Read the model definition and answer for the solid it produces. Units are mm, in the model's axes. Give positions to 0.01 mm unless a question says otherwise; leave off trailing zeros. Loops run counter-clockwise (first coordinate to the right, second up) from the corner with the lowest first, then second, coordinate; pieces in that order, holes last. Notation, with made-up numbers: (15.25, -32.5) - (50.25, -32.5) arc R16 ccw to (50.25, -28.5) - close; hole circle Ø5 at (-30, -28). An arc over 180 degrees is marked (long way). Write item = value, one per line. Start each with the question number.
Autodesk Inventor part; units mm, degrees
ref_plane "YZ Plane" through (0, 0, 0) normal (1, 0, 0) x (0, 1, 0)
ref_plane "XZ Plane" through (0, 0, 0) normal (0, 1, 0) x (-1, 0, 0)
ref_plane "XY Plane" through (0, 0, 0) normal (0, 0, 1) x (1, 0, 0)
sketch "Sketch1" plane through (0, 0, 0) normal (0, 1, 0) x (-1, 0, 0)
  circle A0 centre (0, 0) radius 37.85 construction
  circle A1 centre (0, 0) radius 38.85
  circle A2 centre (0, 0) radius 40.35
  circle A3 centre (0, 0) radius 43.35
  line L0 (1.5, -43.35) -> (-1.5, -43.35)
  line L1 (-1.5, -43.35) -> (-1.5, 0)
  line L2 (-1.5, 0) -> (1.5, 0)
  line L3 (1.5, 0) -> (1.5, -43.35)
  point P0 (0, -43.35)
  point P1 (1.5, -40.3221)
  point P2 (1.5, -38.821)
  point P3 (-1.5, -38.821)
  point P4 (-1.5, -40.3221)
  dimension "d0" = 75.7
  dimension "d1" = 1
  dimension "d2" = 1.5
  dimension "d3" = 3
  dimension "d4" = 3
extrude "Extrusion1" add sketch "Sketch1" along normal blind 10 contours L1 A3 L3 A2 | A2 L3 A3 L1
extrude "Extrusion2" add sketch "Sketch1" along normal blind 10 contours A1 L3 A2 L1 picked at (1.1667, -39.33)
pattern_circular "Circular Pattern1" count 16 over 360 about axis through (0, -10, 0) along (0, 1, 0) of "Extrusion2"
properties part number "STI Hybrid 98 Cooling Shroud Lower Section Prototype_3DPrint"
1. For a pull along X with two mould halves and no side action, classify faces 1 (the flat face through (36, 10, -16)), 2 (the cylindrical face through (-27.486, 4.93, -27.456)) as released by +X, released by -X, zero draft, split by the parting line, or undercut.
2. Given P1, Ø5, axis at y = 1.5, z = 6.5, coming from the +X side; P2, Ø1, axis at y = 4.5, z = -20, coming from the -X side; P3, Ø0.5, axis at x = 39.5, y = 3.5, coming from the -Z side, each flat-ended and moving along its own axis, determine where each tip first touches the part or whether it passes through.
3. A cutting plane is placed at A-A on z = 0. Give the vertices of the cut face in (x, y).
4. Consider line 1 along Z through (x, y) = (-0.5, 7.5); line 2 along Z through (x, y) = (27, 9); line 3 along X through (y, z) = (0.5, 34.5). Determine where each line is inside the solid, lowest interval first. Write a range as [from, to].
5. A cutting plane is placed at B-B on x = 0. Give the vertices of the cut face in (y, z).
Reply:
q1.face_1 = zero draft
q1.face_2 = undercut
q2.P1 = 43.17
q2.P2 = -38.72
q2.P3 = -18.4
q3.outline = (-43.35, 0) - (-38.85, 0) - (-38.85, 10) - (-43.35, 10) - close; (38.85, 0) - (43.35, 0) - (43.35, 10) - (38.85, 10) - close
q4.line_1 = [-43.35, -38.85], [38.85, 43.35]
q4.line_2 = [-33.91, -29.99], [-29.12, -27.93], [27.93, 29.12], [29.99, 33.91]
q4.line_3 = [-26.25, -20.93], [20.93, 26.25]
q5.outline = (0, -43.35) - (10, -43.35) - (10, -38.85) - (0, -38.85) - close; (0, 38.85) - (10, 38.85) - (10, 43.35) - (0, 43.35) - close
